from build123d import *

# Parameters (mm, degrees)
SKETCH1_W                   = 6
SKETCH1_H                   = 50
BOSS_EXTRUDE1_DEPTH         = 42
TAP_DRILL_FOR_M3_TAP1_D     = 2.5
TAP_DRILL_FOR_M3_TAP1_DEPTH = 10
TAP_DRILL_FOR_M3_TAP1_TIP   = 0.751075774
TAP_DRILL_FOR_M3_TAP2_D     = 2.5
TAP_DRILL_FOR_M3_TAP2_DEPTH = 7
TAP_DRILL_FOR_M3_TAP2_TIP   = 0.751075774
SKETCH6_R                   = 18.55
CUT_EXTRUDE1_DEPTH          = 3
CUT_EXTRUDE2_REACH          = 67.368
SKETCH7_R                   = 6.05
SKETCH7_R_2                 = 1.5
CIRPATTERN1_OUTLINE_R       = 1.5
CIRPATTERN1_DEPTH           = 3
CHAMFER1_SIZE               = 1.4


# Read off the part's stored shape, not the designer's step: CirPattern1
with BuildPart() as part:
    # Sketch1 → Boss-Extrude1 (new body)
    with BuildSketch(Plane(origin=(0, 0, 0), x_dir=(1, 0, 0), z_dir=(0, 1, 0))):
        with Locations((3, 25)):
            Rectangle(SKETCH1_W, SKETCH1_H)
    extrude(amount=BOSS_EXTRUDE1_DEPTH)

    # Tap Drill for M3 Tap1
    with Locations(Plane(origin=(0, 42, 0), x_dir=(-1, 0, 0), z_dir=(0, 1, 0))):
        with Locations((-3, -10), (-3, -40)):
            Hole(TAP_DRILL_FOR_M3_TAP1_D / 2, depth=TAP_DRILL_FOR_M3_TAP1_DEPTH)
            with Locations((0, 0, -(TAP_DRILL_FOR_M3_TAP1_DEPTH + TAP_DRILL_FOR_M3_TAP1_TIP / 2))):  # 118° drill point
                Cone(0, TAP_DRILL_FOR_M3_TAP1_D / 2, TAP_DRILL_FOR_M3_TAP1_TIP, mode=Mode.SUBTRACT)

    # Tap Drill for M3 Tap2
    with Locations(Plane.XZ):
        with Locations((3, -10), (3, -40)):
            Hole(TAP_DRILL_FOR_M3_TAP2_D / 2, depth=TAP_DRILL_FOR_M3_TAP2_DEPTH)
            with Locations((0, 0, -(TAP_DRILL_FOR_M3_TAP2_DEPTH + TAP_DRILL_FOR_M3_TAP2_TIP / 2))):  # 118° drill point
                Cone(0, TAP_DRILL_FOR_M3_TAP2_D / 2, TAP_DRILL_FOR_M3_TAP2_TIP, mode=Mode.SUBTRACT)

    # Sketch6 → Cut-Extrude1 (cut)
    with BuildSketch(Plane(origin=(6, 0, 0), x_dir=(0, 0, -1), z_dir=(1, 0, 0))):
        with Locations((25, 19.5)):
            Circle(SKETCH6_R)
    extrude(amount=-CUT_EXTRUDE1_DEPTH, mode=Mode.SUBTRACT)

    # Sketch7 → Cut-Extrude2 (cut, up to next)
    with BuildSketch(Plane(origin=(3, 0, 0), x_dir=(0, 0, -1), z_dir=(1, 0, 0)), mode=Mode.PRIVATE) as cut_extrude2_sk1:
        with Locations((25, 26.5)):
            Circle(SKETCH7_R)
    cut_extrude2_tool1 = extrude(cut_extrude2_sk1.sketch, amount=-CUT_EXTRUDE2_REACH, mode=Mode.PRIVATE) & part.part
    # Sketch7 → Cut-Extrude2 (cut, up to next)
    with BuildSketch(Plane(origin=(3, 0, 0), x_dir=(0, 0, -1), z_dir=(1, 0, 0)), mode=Mode.PRIVATE) as cut_extrude2_sk2:
        with Locations((9.5, 19.5)):
            Circle(SKETCH7_R_2)
    cut_extrude2_tool2 = extrude(cut_extrude2_sk2.sketch, amount=-CUT_EXTRUDE2_REACH, mode=Mode.PRIVATE) & part.part
    add(cut_extrude2_tool1.solids().sort_by_distance((3, 26.5, -25))[0], mode=Mode.SUBTRACT)
    add(cut_extrude2_tool2.solids().sort_by_distance((3, 19.5, -9.5))[0], mode=Mode.SUBTRACT)

    # CirPattern1 outline → CirPattern1 (cut)
    with BuildSketch(Plane.YZ):
        with Locations((32.923393759, -17.25)):
            Circle(CIRPATTERN1_OUTLINE_R)
        with Locations((32.923393759, -32.75)):
            Circle(CIRPATTERN1_OUTLINE_R)
        with Locations((19.5, -40.5)):
            Circle(CIRPATTERN1_OUTLINE_R)
        with Locations((6.076606241, -32.75)):
            Circle(CIRPATTERN1_OUTLINE_R)
        with Locations((6.076606241, -17.25)):
            Circle(CIRPATTERN1_OUTLINE_R)
    extrude(amount=CIRPATTERN1_DEPTH, mode=Mode.SUBTRACT)

    # Chamfer1
    chamfer1_edges = [part.edges().sort_by_distance(p)[0] for p in [
        (0, 19.5, -8),
        (0, 4.576606241, -17.25),
        (0, 4.576606241, -32.75),
        (0, 18, -40.5),
        (0, 31.423393759, -32.75),
        (0, 31.423393759, -17.25),
    ]]
    chamfer(chamfer1_edges, length=CHAMFER1_SIZE)


solid = part.part
Check sheet for the modelled part. Datum: model origin and axes. Units: mm. A direction names the side the tool comes from. Round coordinates to 2 decimals unless told otherwise and drop trailing zeros. Order: outer loops, then holes, each group sorted by start corner. A loop starts at its lowest first (then second) coordinate and runs counter-clockwise, first axis right, second up.
(1) Scan lines: probe 1 along Z at (x, y) = (3.5, 6); probe 2 along X at (y, z) = (4, -40); probe 3 along Y at (x, z) = (4.45, -25). Record each from-to range of solid material in increasing order.
(2) Cross-section at D-D, the plane z = -17.25. Enter the section's corners in (x, y).
(3) Draft check along Y on faces 1 (the conical face through (2.972, 7.621, -39.785)), 2 (the flat face through (6, 35, -14)), 3 (the cylindrical face through (2.19, 6.77, -34.08)). Enter one of: pulls with the +Y half, pulls with the -Y half, needs draft (parallel to the pull), parting line crosses it, or undercut.
(4) Cross-section at B-B, the plane z = -25. Enter the section's corners in (x, y).
(5) Cross-section at C-C, the plane y = 26.5. Enter the section's corners in (x, z).
(6) Cross-section at A-A, the plane y = 19.5. Enter the section's corners in (x, z), and give its area (3 significant figures).
(7) Go/stop test with flat-tipped pins: P1, Ø1.8, axis at y = 19.5, z = -40.5, coming from the +X side (1 decimal); P2, Ø4, axis at y = 19.5, z = -9.5, coming from the -X side; P3, Ø3.5, axis at y = 6.08, z = -32.75, coming from the -X side; P4, Ø2, axis at x = 3, z = -40, coming from the -Y side. Record where each tip stops, or that it passes through.
(8) Access from +Z, -Z, +X, -X, +Y, -Y to the whole of each face (thin tool, end or side, straight path). Record for faces 4 (the cylindrical face through (3.672, 36.93, -8.946)), 5 (the cylindrical face through (2.328, 3.549, -8.946)), 6 (the cylindrical face through (4.521, 37.892, -22.585)).
Check sheet entries:
1. probe 1: z = -50 to -41.15, -38.85 to -37.72, -12.28 to -11.15, -8.85 to 0
1. probe 2: x = 0 to 1.75, 4.25 to 6
1. probe 3: y = 0 to 0.95, 38.05 to 42
2. outline: (0, 0) - (6, 0) - (6, 2.65) - (3, 2.65) - (3, 4.58) - (1.4, 4.58) - (0, 3.18) - close; (0, 8.98) - (1.4, 7.58) - (3, 7.58) - (3, 31.42) - (1.4, 31.42) - (0, 30.02) - close; (0, 35.82) - (1.4, 34.42) - (3, 34.42) - (3, 36.35) - (6, 36.35) - (6, 42) - (0, 42) - close
3. face 1: pulls with the -Y half
3. face 2: needs draft
3. face 3: undercut
4. outline: (0, 0) - (6, 0) - (6, 0.95) - (3, 0.95) - (3, 20.45) - (0, 20.45) - close; (0, 32.55) - (3, 32.55) - (3, 38.05) - (6, 38.05) - (6, 42) - (0, 42) - close
5. outline: (0, -50) - (6, -50) - (6, -42.18) - (3, -42.18) - (3, -31.05) - (0, -31.05) - close; (0, -18.95) - (3, -18.95) - (3, -7.82) - (6, -7.82) - (6, 0) - (0, 0) - close
6. outline: (0, -50) - (6, -50) - (6, -43.55) - (3, -43.55) - (3, -42) - (1.4, -42) - (0, -43.4) - close; (0, -37.6) - (1.4, -39) - (3, -39) - (3, -11) - (1.4, -11) - (0, -12.4) - close; (0, -6.6) - (1.4, -8) - (3, -8) - (3, -6.45) - (6, -6.45) - (6, 0) - (0, 0) - close
6. area: 167 mm2
7. P1: passes through
7. P2: stops at x = 0.9
7. P3: stops at x = 1.15
7. P4: stops at y = 7.15
8. face 4: +Y
8. face 5: -Y
8. face 6: +X
